Source: CAD feature listing. Evaluate the final solid. Frame: model axes, mm. A direction names the side the tool comes from. Give positions to 0.01 mm unless a question says otherwise; leave off trailing zeros. Order: outer loops, then holes, each group sorted by start corner. A loop starts at its lowest first (then second) coordinate and runs counter-clockwise, first axis right, second up. Notation, with made-up numbers: (-15, 19) -> (16, 19) arc R23 cw to (16, 53) -> close; hole circle Ø6 at (47, 36). An arc over 180 degrees is marked (long way). Answer in a Markdown table with one row per item.
```python
from build123d import *

# Parameters (mm, degrees)
SKETCH1_W                           = 60
SKETCH1_H                           = 10
BOSS_EXTRUDE1_DEPTH                 = 40
M3X0_5_TAPPED_HOLE3_D               = 2.5
M3X0_5_TAPPED_HOLE3_DEPTH           = 10
M3X0_5_TAPPED_HOLE3_TIP             = 0.751075774
M3X0_5_TAPPED_HOLE2_D               = 2.5
M3X0_5_TAPPED_HOLE2_DEPTH           = 5
M3X0_5_TAPPED_HOLE2_TIP             = 0.751075774
M3X0_5_TAPPED_HOLE2_ON_FACE_2_D     = 2.5
M3X0_5_TAPPED_HOLE2_ON_FACE_2_DEPTH = 5
M3X0_5_TAPPED_HOLE2_ON_FACE_2_TIP   = 0.751075774


with BuildPart() as part:
    # Sketch1 → Revolve1 (revolve)
    with BuildSketch(Plane.XY):
        with Locations((30, 5)):
            Rectangle(SKETCH1_W, SKETCH1_H)
    revolve(axis=Axis((0, 0, 0), (1, 0, 0)))

    # Sketch3 → Boss-Extrude1 (add)
    with BuildSketch(Plane(origin=(60, 0, 0), x_dir=(0, 0, -1), z_dir=(1, 0, 0))):
        with BuildLine():
            Line((-6.614378278, -7.5), (-6.614378278, 7.5))
            ThreePointArc((-6.614378278, 7.5), (0, 10), (6.614378278, 7.5))
            Line((6.614378278, 7.5), (6.614378278, -7.5))
            ThreePointArc((6.614378278, -7.5), (0, -10), (-6.614378278, -7.5))
        make_face()
    extrude(amount=BOSS_EXTRUDE1_DEPTH)

    # M3x0.5 Tapped Hole3
    with Locations(Plane.XY.offset(10)):
        with Locations((30, 0)):
            Hole(M3X0_5_TAPPED_HOLE3_D / 2, depth=M3X0_5_TAPPED_HOLE3_DEPTH)
            with Locations((0, 0, -(M3X0_5_TAPPED_HOLE3_DEPTH + M3X0_5_TAPPED_HOLE3_TIP / 2))):  # 118° drill point
                Cone(0, M3X0_5_TAPPED_HOLE3_D / 2, M3X0_5_TAPPED_HOLE3_TIP, mode=Mode.SUBTRACT)

    # M3x0.5 Tapped Hole2
    with Locations(Plane(origin=(70, 0, 6.614378278), x_dir=(1, 0, 0), z_dir=(0, 0, 1))):
        with Locations((0, 0), (15, 0)):
            Hole(M3X0_5_TAPPED_HOLE2_D / 2, depth=M3X0_5_TAPPED_HOLE2_DEPTH)
            with Locations((0, 0, -(M3X0_5_TAPPED_HOLE2_DEPTH + M3X0_5_TAPPED_HOLE2_TIP / 2))):  # 118° drill point
                Cone(0, M3X0_5_TAPPED_HOLE2_D / 2, M3X0_5_TAPPED_HOLE2_TIP, mode=Mode.SUBTRACT)

    # M3x0.5 Tapped Hole2 on face 2
    with Locations(Plane(origin=(85, 0, -6.614378278), x_dir=(-1, 0, 0), z_dir=(0, 0, -1))):
        with Locations((0, 0), (15, 0)):
            Hole(M3X0_5_TAPPED_HOLE2_ON_FACE_2_D / 2, depth=M3X0_5_TAPPED_HOLE2_ON_FACE_2_DEPTH)
            with Locations((0, 0, -(M3X0_5_TAPPED_HOLE2_ON_FACE_2_DEPTH + M3X0_5_TAPPED_HOLE2_ON_FACE_2_TIP / 2))):  # 118° drill point
                Cone(0, M3X0_5_TAPPED_HOLE2_ON_FACE_2_D / 2, M3X0_5_TAPPED_HOLE2_ON_FACE_2_TIP, mode=Mode.SUBTRACT)


solid = part.part
```
(1) Pull-direction query (Y, two-part tool) for faces 6 (the cylindrical face through (38.189, 9.227, -3.856)), 7 (the conical face through (85.17, -0.13, -0.99)), 8 (the flat face through (80, 0, 6.614)); classes: +Y half, -Y half, draft (parallel to the pull), parting line (faces both ways), or undercut.
A:
| item | result |
|---|---|
| face 6 | parting line |
| face 7 | undercut |
| face 8 | draft |
(2) Section query C-C (x = 72.5). Return the cut outline in (y, z).
A:
| item | result |
|---|---|
| outline | (-7.5, -6.61) -> (7.5, -6.61) arc R10 ccw to (7.5, 6.61) -> (-7.5, 6.61) arc R10 ccw to start |
(3) Section query B-B (z = 3.75). Return the cut outline in (x, y), plus the area to 3 significant figures.
A:
| item | result |
|---|---|
| outline | (0, -9.27) -> (100, -9.27) -> (100, 9.27) -> (0, 9.27) -> close; hole circle Ø2.5 at (30, 0); hole circle Ø2.5 at (70, 0); hole circle Ø2.5 at (85, 0) |
| area | 1,840 mm^2 |
(4) Ray query, probe 1 along X at (y, z) = (0, 4); probe 2 along X at (y, z) = (0, -3.7); probe 3 along X at (y, z) = (0.75, 4.25). Return the intervals inside material, ascending.
A:
| item | result |
|---|---|
| probe 1 | x = 0 to 28.75, 31.25 to 68.75, 71.25 to 83.75, 86.25 to 100 |
| probe 2 | x = 0 to 68.75, 71.25 to 83.75, 86.25 to 100 |
| probe 3 | x = 0 to 29, 31 to 69, 71 to 84, 86 to 100 |
(5) Section query A-A (y = -6). Return the cut outline in (x, z), plus the area to 3 significant figures.
A:
| item | result |
|---|---|
| outline | (0, -8) -> (60, -8) -> (60, -6.61) -> (100, -6.61) -> (100, 6.61) -> (60, 6.61) -> (60, 8) -> (0, 8) -> close |
| area | 1,490 mm^2 |
(6) Access query for faces 1 (the cylindrical face through (86.19, 0.38, -4.08)), 2 (the cylindrical face through (83.81, 0.38, 4.08)), 3 (the flat face through (80, 0, -6.614)), 4 (the flat face through (0, 0, 0)), 5 (the flat face through (60, 0, 8)). Directions: +Z, -Z, +X, -X, +Y, -Y. A direction counts if a zero-diameter tool reaches every point of the face in a straight line with its end or side. Return the directions, or none.
A:
| item | result |
|---|---|
| face 1 | -Z |
| face 2 | +Z |
| face 3 | -Z, +X, +Y, -Y |
| face 4 | +Z, -Z, -X, +Y, -Y |
| face 5 | +Z, +X, +Y, -Y |
(7) Section query D-D (z = -5). Return the cut outline in (x, y), plus the area to 3 significant figures.
A:
| item | result |
|---|---|
| outline | (0, -8.66) -> (100, -8.66) -> (100, 8.66) -> (0, 8.66) -> close; hole circle Ø2.5 at (70, 0); hole circle Ø2.5 at (85, 0) |
| area | 1,720 mm^2 |
(8) First-contact query: pin 1 Ø3 at (x, y) = (85, 0) entering from +Z; pin 2 Ø2 at (x, y) = (70, 0) entering from -Z; pin 3 Ø8 at (x, z) = (54.5, 7) entering from +Y. Flat tips, straight axial feed; report the tip coordinate or a pass-through.
A:
| item | result |
|---|---|
| pin 1 | stops at z = 6.61 |
| pin 2 | stops at z = -1.46 |
| pin 3 | stops at y = 9.54 |
